from build123d import *

# Parameters (mm, degrees)
SKETCH_R     = 1.05
PAD_DEPTH    = 3.5
SKETCH001_R  = 15
PAD001_DEPTH = 7
SKETCH002_R  = 1
POCKET_DEPTH = 10


with BuildPart() as part:
    # Sketch → Pad (new body)
    with BuildSketch(Plane.XY):
        with BuildLine():
            ThreePointArc((0, 15), (-14.003706, -5.375519), (10.036959, -11.147172))
            Line((10.036959, -11.147172), (20, -2.17641))
            Line((20, -2.17641), (28.298795, -5))
            ThreePointArc((28.298795, -5), (35, -1.701205), (31.701205, 5))
            Line((2.310268, 15), (31.701205, 5))
            Line((0, 15), (2.310268, 15))
        make_face()
        with Locations((30, 0)):
            Circle(SKETCH_R, mode=Mode.SUBTRACT)
    extrude(amount=PAD_DEPTH)

    # Sketch001 → Pad001 (join)
    with BuildSketch(Plane.XY):
        Circle(SKETCH001_R)
    extrude(amount=PAD001_DEPTH)

    # Sketch002 → Pocket (cut)
    with BuildSketch(Plane.XY):
        with Locations((-5.656854, 5.656854)):
            Circle(SKETCH002_R)
        with Locations((5.656854, 5.656854)):
            Circle(SKETCH002_R)
        with Locations((5.656854, -5.656854)):
            Circle(SKETCH002_R)
        with Locations((-5.656854, -5.656854)):
            Circle(SKETCH002_R)
    extrude(amount=POCKET_DEPTH, mode=Mode.SUBTRACT)


solid = part.part
CAD build for the part. Positions are in the model's coordinates, mm. A direction names the side the tool comes from. Give positions to 0.01 mm unless a question says otherwise; leave off trailing zeros. Write each loop counter-clockwise with the first axis right and the second up, starting at its lowest first coordinate (ties: lowest second). Pieces come first, ordered by that corner, then holes. Notation, with made-up numbers: (-36.75, -33) - (-3.75, -33) arc R34 ccw to (-3.75, 2) - close; hole circle Ø8 at (57.25, 44.5). An arc over 180 degrees is marked (long way). Put each result on its own line as item: value.
(1) Saw through at A-A (y = 0). List the corners of the cut face in (x, z), then the cut area to 3 significant figures.
Working result:
outline: (-15, 0) - (28.95, 0) - (28.95, 3.5) - (15, 3.5) - (15, 7) - (-15, 7) - close; (31.05, 0) - (35.28, 0) - (35.28, 3.5) - (31.05, 3.5) - close
area: 274 mm^2
(2) Wall check: L1, parallel to Y at x = 6, z = 0.5; L2, parallel to Y at x = -6.5, z = 1.25; L3, parallel to Z at x = 24, y = 6. Give the ranges that are in metal, low to high.
Working result:
L1: -13.75 to -6.6, -4.72 to 4.72, 6.6 to 13.75
L2: -13.52 to -6.19, -5.12 to 5.12, 6.19 to 13.52
L3: 0 to 3.5
(3) Tool access for faces 4 (the flat face through (24.09, -3.57, 1.73)), 5 (the cylindrical face through (-12, -9, 3)), 6 (the flat face through (1, 15, 2)): list every direction of +Z, -Z, +X, -X, +Y, -Y with a clear straight run to the whole face (end or side of a thin tool).
Working result:
face 4: +Z, -Z, -Y
face 5: +Z
face 6: +Z, -Z, +X, -X, +Y
(4) Saw through at C-C (z = 1.75). List the corners of the cut face in (x, y).
Working result:
outline: (0, 15) arc R15 ccw (long way) to (10.04, -11.15) - (20, -2.18) - (28.3, -5) arc R5.28 ccw to (31.7, 5) - (6.03, 13.73) arc R15 ccw to (3.6, 14.56) - (2.31, 15) - close; hole circle Ø2 at (-5.66, -5.66); hole circle Ø2 at (-5.66, 5.66); hole circle Ø2 at (5.66, -5.66); hole circle Ø2 at (5.66, 5.66); hole circle Ø2.1 at (30, 0)
(5) Saw through at D-D (x = 5.5). List the corners of the cut face in (y, z), then the cut area to 3 significant figures.
Working result:
outline: (-13.96, 0) - (-6.64, 0) - (-6.64, 7) - (-13.96, 7) - close; (-4.67, 0) - (4.67, 0) - (4.67, 7) - (-4.67, 7) - close; (6.64, 0) - (13.96, 0) - (13.96, 7) - (6.64, 7) - close
area: 168 mm^2
(6) Drop flat-ended pins along their axis: pin 1 Ø3 at (x, z) = (14.5, 2.5) entering from -Y; pin 2 Ø3 at (x, z) = (-8, 3.5) entering from -Y; pin 3 Ø2 at (y, z) = (5, 5.5) entering from -X; pin 4 Ø1.6 at (x, y) = (-5.66, -5.66) entering from -Z. Give the stop position or say it passes through.
Working result:
pin 1: y = -8.48
pin 2: y = -13.52
pin 3: x = -14.46
pin 4: through
(7) Saw through at B-B (x = 30). List the corners of the cut face in (y, z), then the cut area to 3 significant figures.
Working result:
outline: (-5.28, 0) - (-1.05, 0) - (-1.05, 3.5) - (-5.28, 3.5) - close; (1.05, 0) - (5.58, 0) - (5.58, 3.5) - (1.05, 3.5) - close
area: 30.7 mm^2
(8) Pull direction Y, two halves, no side cores. Call faces 1 (the flat face through (0, 0, 7)), 2 (the flat face through (14.95, -6.723, 1.726)), 3 (the cylindrical face through (4.92, 6.33, 3.45)): released by +Y, released by -Y, zero draft, split by the parting line, or undercut.
Working result:
face 1: zero draft
face 2: released by -Y
face 3: undercut
